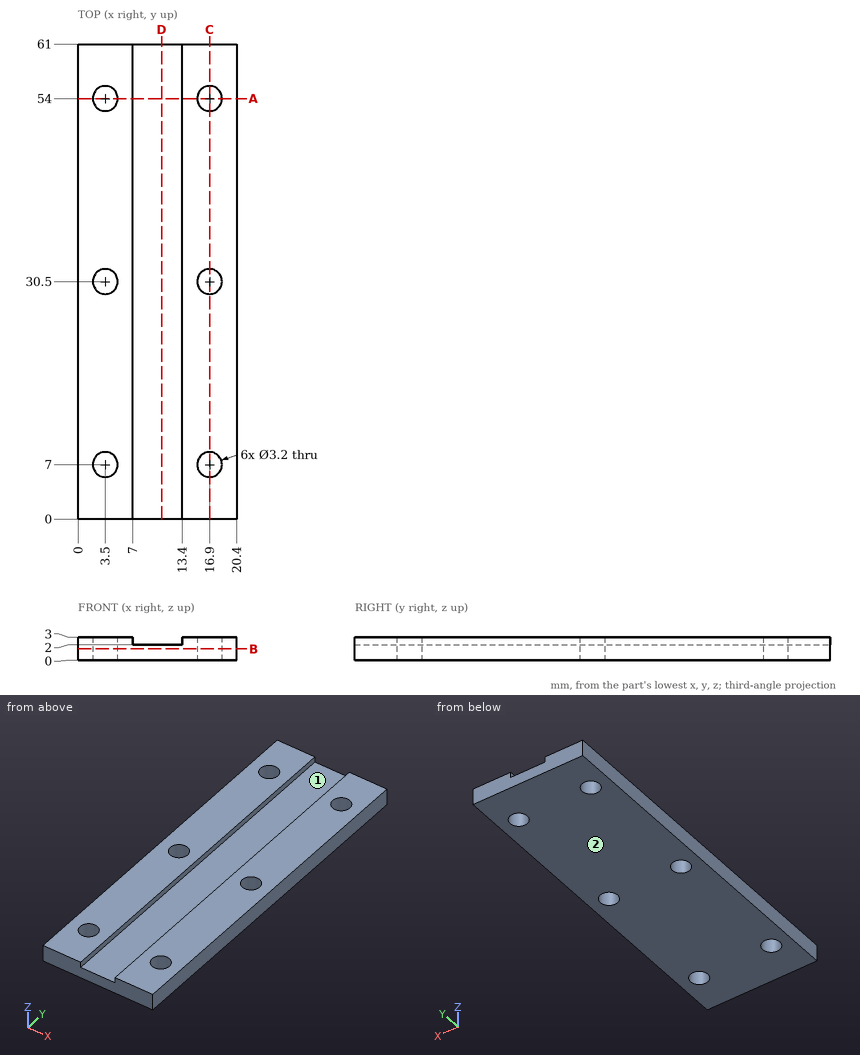
Geometry: see drawing. Coordinates: mm, zero at the bounding-box minimum. A direction names the side the tool comes from. Round coordinates to 2 decimals unless told otherwise and drop trailing zeros. Order: outer loops, then holes, each group sorted by start corner. A loop starts at its lowest first (then second) coordinate and runs counter-clockwise, first axis right, second up. Notation, with made-up numbers: (-23.75, 39) -> (29.25, 39) arc R17 cw to (29.25, 58) -> close; hole circle Ø2 at (42, 42). An arc over 180 degrees is marked (long way). Use CSV: the item, a comma, the result in double quotes.
(1) First-contact query: pin 1 Ø5 at (x, y) = (10, 24) entering from +Z. Flat tip, straight axial feed; report the tip coordinate or a pass-through.
Report:
pin 1,"z = 2"
(2) Section C-C on x = 16.9. Return the cut outline in (y, z), and give its area (3 significant figures).
Report:
outline,"(0, 0) -> (5.4, 0) -> (5.4, 3) -> (0, 3) -> close; (8.6, 0) -> (28.9, 0) -> (28.9, 3) -> (8.6, 3) -> close; (32.1, 0) -> (52.4, 0) -> (52.4, 3) -> (32.1, 3) -> close; (55.6, 0) -> (61, 0) -> (61, 3) -> (55.6, 3) -> close"
area,"154 mm^2"
(3) Access query for the marked faces 1 and 2. Directions: +Z, -Z, +X, -X, +Y, -Y. A direction counts if a zero-diameter tool reaches every point of the face in a straight line with its end or side. Return the directions, or none.
Report:
face 1,"+Z, +Y, -Y"
face 2,"-Z, +X, -X, +Y, -Y"
(4) Section B-B on z = 1.5. Return the cut outline in (x, y), and give its area (3 significant figures).
Report:
outline,"(0, 0) -> (20.4, 0) -> (20.4, 61) -> (0, 61) -> close; hole circle Ø3.2 at (3.5, 7); hole circle Ø3.2 at (3.5, 30.5); hole circle Ø3.2 at (3.5, 54); hole circle Ø3.2 at (16.9, 7); hole circle Ø3.2 at (16.9, 30.5); hole circle Ø3.2 at (16.9, 54)"
area,"1,200 mm^2"
(5) Section A-A on y = 54. Return the cut outline in (x, z), and give its area (3 significant figures).
Report:
outline,"(0, 0) -> (1.9, 0) -> (1.9, 3) -> (0, 3) -> close; (5.1, 0) -> (15.3, 0) -> (15.3, 3) -> (13.4, 3) -> (13.4, 2) -> (7, 2) -> (7, 3) -> (5.1, 3) -> close; (18.5, 0) -> (20.4, 0) -> (20.4, 3) -> (18.5, 3) -> close"
area,"35.6 mm^2"
(6) Ray query, L1, parallel to Y at x = 3.5, z = 1.7; L2, parallel to X at y = 46.5, z = 2.6; L3, parallel to Z at x = 12, y = 32.5. Return the intervals inside material, ascending.
Report:
L1,"0 to 5.4, 8.6 to 28.9, 32.1 to 52.4, 55.6 to 61"
L2,"0 to 7, 13.4 to 20.4"
L3,"0 to 2"
(7) Section D-D on x = 10.75. Return the cut outline in (y, z).
Report:
outline,"(0, 0) -> (61, 0) -> (61, 2) -> (0, 2) -> close"
